from build123d import *

# Parameters (mm, degrees)
CROQUIS1_W              = 7.7
CROQUIS1_H              = 7.7
SALIENTE_EXTRUIR1_DEPTH = 2.5
CROQUIS2_R              = 1.4
SALIENTE_EXTRUIR2_DEPTH = 7.5
CROQUIS6_R              = 0.6
CORTAR_EXTRUIR1_DEPTH   = 19.327438542


with BuildPart() as part:
    # Croquis1 → Saliente-Extruir1 (new body)
    with BuildSketch(Plane.XY):
        Rectangle(CROQUIS1_W, CROQUIS1_H)
    extrude(amount=SALIENTE_EXTRUIR1_DEPTH)

    # Croquis2 → Saliente-Extruir2 (add)
    with BuildSketch(Plane(origin=(0, 0, 0), x_dir=(-1, 0, 0), z_dir=(0, 0, -1))):
        Circle(CROQUIS2_R)
    saliente_extruir2 = extrude(amount=SALIENTE_EXTRUIR2_DEPTH)

    # Recubrir2: read off the stored shape, not the designer's step
    # Recubrir2: loft between two sections, ruled curve by curve
    recubrir2_from = [
        Edge.make_bspline([(-0.33839724, 1.767904779, -2.5), (3.197412318, 2.44469926, -2.5), (3.874206798, -1.091110298, -2.5), (0.33839724, -1.767904779, -2.5), (-3.197412318, -2.44469926, -2.5), (-3.874206798, 1.091110298, -2.5), (-0.33839724, 1.767904779, -2.5)], [0, 0, 0, 0, 0.5, 0.5, 0.5, 1, 1, 1, 1], 3, [1, 0.333333333, 0.333333333, 1, 0.333333333, 0.333333333, 1]),
    ]
    recubrir2_to = [
        Edge.make_bspline([(-0.867767345, 1.09862634, -6), (1.329485334, 2.83416103, -6), (3.065020025, 0.636908351, -6), (0.867767345, -1.09862634, -6), (-1.329485334, -2.83416103, -6), (-3.065020025, -0.636908351, -6), (-0.867767345, 1.09862634, -6)], [0, 0, 0, 0, 0.5, 0.5, 0.5, 1, 1, 1, 1], 3, [1, 0.333333333, 0.333333333, 1, 0.333333333, 0.333333333, 1]),
    ]
    recubrir2 = Solid(Shell([*[Face.make_surface_from_curves(recubrir2_from[k], recubrir2_to[k]) for k in range(1)], Face(Wire(recubrir2_from)), Face(Wire(recubrir2_to))]))
    add(recubrir2)

    # Simetría2: Saliente-Extruir2, Recubrir2 across plane
    add(saliente_extruir2.mirror(Plane(origin=(0, 0, 1.25), x_dir=(1, 0, 0), z_dir=(0, 0, -1))))
    add(recubrir2.mirror(Plane(origin=(0, 0, 1.25), x_dir=(1, 0, 0), z_dir=(0, 0, -1))))

    # Croquis6 → Cortar-Extruir1 (cut, through all)
    with BuildSketch(Plane(origin=(0, 0, -7.5), x_dir=(-1, 0, 0), z_dir=(0, 0, -1))):
        Circle(CROQUIS6_R)
    extrude(amount=-CORTAR_EXTRUIR1_DEPTH, mode=Mode.SUBTRACT)


solid = part.part
Check sheet for the modelled part. Datum: model origin and axes. Units: mm. A direction names the side the tool comes from. Round coordinates to 2 decimals unless told otherwise and drop trailing zeros. Loops run counter-clockwise (first coordinate to the right, second up) from the corner with the lowest first, then second, coordinate; pieces in that order, holes last. Notation, with made-up numbers: (54.25, -8) -> (81.25, -8) arc R31 cw to (81.25, 27) -> close; hole circle Ø1 at (8, 57). An arc over 180 degrees is marked (long way). Put each result on its own line as item: value. Start each with the question number.
1. Gauge pin test, flat ends, axial feed: pin 1 (1.5 mm diameter, centred on x = -1, y = -2.5, fed in from +Z); pin 2 (2 mm diameter, centred on x = -1.5, z = -2, fed in from +Y); pin 3 (1 mm diameter, centred on x = 2, z = 3.5, fed in from -Y). Record the tip position at first contact, or that the pin passes through.
2. Section check A-A (z = 1.25). Enter the section's corners in (x, y), plus the area to 3 significant figures.
3. Draft check along X on faces 1 (the face through (3.85, 0, 1)), 2 (the face through (1.4, 0.06, 3.73)), 3 (the face through (-0.323, 0.506, 1.127)). Enter one of: +X half, -X half, draft (parallel to the pull), parting line (faces both ways), or undercut.
4. Scan lines: probe 1 along Z at (x, y) = (3, 3.5); probe 2 along Y at (x, z) = (0, -2); probe 3 along Y at (x, z) = (0, -4). Record each from-to range of solid material in increasing order.
5. Section check B-B (x = 2.5). Enter the section's corners in (y, z).
6. Access from +Z, -Z, +X, -X, +Y, -Y to the whole of each face (thin tool, end or side, straight path). Record for faces 4 (the face through (1.4, 0.06, -1.23)), 5 (the face through (-3.85, 0, 1)), 6 (the face through (-1.335, 0.421, -6.739)), 7 (the face through (-1.335, 0.421, 9.239)).
Findings:
1. pin 1: stops at z = 2.5
1. pin 2: stops at y = 1.68
1. pin 3: passes through
2. outline: (-3.85, -3.85) -> (3.85, -3.85) -> (3.85, 3.85) -> (-3.85, 3.85) -> close; hole circle Ø1.2 at (0, 0)
2. area: 58.2 mm^2
3. face 1: +X half
3. face 2: parting line
3. face 3: undercut
4. probe 1: z = 0 to 2.5
4. probe 2: y = -1.4 to -0.6, 0.6 to 1.4
4. probe 3: y = -1.59 to -0.6, 0.6 to 1.59
5. outline: (-3.85, 0) -> (3.85, 0) -> (3.85, 2.5) -> (-3.85, 2.5) -> close
6. face 4: none
6. face 5: +Z, -Z, -X, +Y, -Y
6. face 6: -Z
6. face 7: +Z
